The listing builds one solid part. Answer for the finished solid, in the listing's coordinates (mm). A direction names the side the tool comes from. Give positions to 0.01 mm unless a question says otherwise; leave off trailing zeros. Write each loop counter-clockwise with the first axis right and the second up, starting at its lowest first coordinate (ties: lowest second). Pieces come first, ordered by that corner, then holes. Notation, with made-up numbers: (86.25, 73) - (141.25, 73) arc R16 ccw to (141.25, 77) - close; hole circle Ø1 at (27.5, 73). An arc over 180 degrees is marked (long way). Use a Markdown table: item, result. Add a question column.
from build123d import *

# Parameters (mm, degrees)
SKETCH2_R          = 1.6
CUT_EXTRUDE1_DEPTH = 2
CUT_EXTRUDE3_DEPTH = 9
CIRPATTERN1_COUNT  = 3
SKETCH5_R          = 2.45
CUT_EXTRUDE4_DEPTH = 8.5
SKETCH6_R          = 0.5
CUT_EXTRUDE5_DEPTH = 8.5
CUT_EXTRUDE6_DEPTH = 8.5


with BuildPart() as part:
    # Sketch1 → Revolve1 (revolve)
    with BuildSketch(Plane.XY):
        with BuildLine():
            Line((0, -13.977445887), (3.15, -13.977445887))
            ThreePointArc((3.15, -13.977445887), (3.220710678, -14.006735209), (3.25, -14.077445887))
            Line((3.25, -14.077445887), (3.25, -15.377445887))
            Line((3.25, -15.377445887), (3.4, -15.377445887))
            ThreePointArc((3.4, -15.377445887), (4.602081528, -15.875364359), (5.1, -17.077445887))
            Line((5.1, -17.077445887), (5.1, -22.177445887))
            ThreePointArc((5.1, -22.177445887), (4.602081528, -23.379527415), (3.4, -23.877445887))
            Line((3.4, -23.877445887), (3.35, -23.877445887))
            Line((3.35, -23.877445887), (3.35, -24.877445887))
            ThreePointArc((3.35, -24.877445887), (3.320710678, -24.948156565), (3.25, -24.977445887))
            Line((3.25, -24.977445887), (0, -24.977445887))
            Line((0, -24.977445887), (0, -13.977445887))
        make_face()
    revolve(axis=Axis((0, 36.866666667, 0), (0, -1, 0)))

    # Sketch2 → Cut-Extrude1 (cut)
    with BuildSketch(Plane(origin=(0, -13.977445887, 0), x_dir=(1, 0, 0), z_dir=(0, 1, 0))):
        Circle(SKETCH2_R)
    extrude(amount=-CUT_EXTRUDE1_DEPTH, mode=Mode.SUBTRACT)

    # Sketch4 → Cut-Extrude3 (cut)
    with BuildSketch(Plane(origin=(0, -15.977445887, 0), x_dir=(1, 0, 0), z_dir=(0, 1, 0))):
        with BuildLine():
            Line((-0.42, 0.319853318), (-0.42, 1.543891188))
            ThreePointArc((-0.42, 1.543891188), (-1.354595532, 0.832929416), (-1.539787712, -0.326656419))
            Line((-1.539787712, -0.326656419), (-0.42, 0.319853318))
        make_face()
    cut_extrude3 = extrude(amount=-CUT_EXTRUDE3_DEPTH, mode=Mode.SUBTRACT)

    # CirPattern1: Cut-Extrude3 ×3 about axis
    cirpattern1_axis = Axis((0, 0, -0.022012107), (0, 1, 0))
    for i in range(1, CIRPATTERN1_COUNT):
        add(cut_extrude3.rotate(cirpattern1_axis, i * 360 / CIRPATTERN1_COUNT), mode=Mode.SUBTRACT)

    # Sketch5 → Cut-Extrude4 (cut)
    with BuildSketch(Plane.XZ.offset(24.977445887)):
        Circle(SKETCH5_R)
    extrude(amount=-CUT_EXTRUDE4_DEPTH, mode=Mode.SUBTRACT)

    # Sketch6 → Cut-Extrude5 (cut)
    with BuildSketch(Plane(origin=(0, 0, 0), x_dir=(0, 0, -1), z_dir=(1, 0, 0))):
        with Locations((-2.1, -18.477445887)):
            Circle(SKETCH6_R)
        with Locations((2.1, -18.477445887)):
            Circle(SKETCH6_R)
    extrude(amount=-CUT_EXTRUDE5_DEPTH, mode=Mode.SUBTRACT)

    # Sketch7 → Cut-Extrude6 (cut)
    with BuildSketch(Plane(origin=(0, 0, 0), x_dir=(0, 0, -1), z_dir=(1, 0, 0))):
        with BuildLine():
            Line((1.502497593, -21.270117784), (-1.5, -21.270117784))
            ThreePointArc((-1.5, -21.270117784), (-1.846335949, -20.923781835), (-1.5, -20.577445887))
            Line((-1.5, -20.577445887), (1.502497593, -20.577445887))
            ThreePointArc((1.502497593, -20.577445887), (1.848833542, -20.923781835), (1.502497593, -21.270117784))
        make_face()
    extrude(amount=-CUT_EXTRUDE6_DEPTH, mode=Mode.SUBTRACT)


solid = part.part
1. The part is cut by section A-A (y = -15). Give the vertices of the cut face in (x, z), and give its area (3 significant figures).
2. Consider L1, parallel to Z at x = 0, y = -21.5; L2, parallel to Y at x = -0.25, z = -1.25. Determine where each line is inside the solid, lowest interval first. Write a range as [from, to].
3. Given P1, Ø5.5, axis at x = 0, z = 0.5, coming from the -Y side; P2, Ø1.5, axis at x = 3.5, y = -23.5, coming from the -Z side; P3, Ø1.5, axis at x = 4, y = -17, coming from the +Z side; P4, Ø3, axis at x = 0, z = 0, coming from the -Y side, each flat-ended and moving along its own axis, determine where each tip first touches the part or whether it passes through.
4. For a pull along X with two mould halves and no side action, classify faces 1 (the cylindrical face through (-3.347, -24.384, 0.147)), 2 (the cylindrical face through (-2.93, -18.67, -2.56)), 3 (the cylindrical face through (2.337, -20.787, 0.736)) as released by +X, released by -X, zero draft, split by the parting line, or undercut.
5. The part is cut by section C-C (y = -23.25). Give the vertices of the cut face in (x, z).
6. The part is cut by section B-B (z = 0). Count the separate pieces of the cut face and the enclosed holes in it, and give its area (3 significant figures).
7. Which of the six approach directions +Z, -Z, +X, -X, +Y, -Y give full straight-line access (tool end or side, diameter ignored) to faces 4 (the flat face through (0, -16.477, 0)), 5 (the cylindrical face through (-2.579, -14.737, -1.978)), 6 (the cylindrical face through (-2.9, -18.5, 2.6))?
Check values:
| question | item | result |
|---|---|---|
| 1 | outline | circle Ø6.5 at (0, 0); hole circle Ø3.2 at (0, 0) |
| 1 | area | 25.1 mm2 |
| 2 | L1 | z = [-5.1, -2.45], [2.45, 5.1] |
| 2 | L2 | y = [-16.48, -15.98] |
| 3 | P1 | stops at y = -24.98 |
| 3 | P2 | stops at z = -3.9 |
| 3 | P3 | stops at z = 3.93 |
| 3 | P4 | stops at y = -16.48 |
| 4 | face 1 | split by the parting line |
| 4 | face 2 | zero draft |
| 4 | face 3 | undercut |
| 5 | outline | circle Ø9.44 at (0, 0); hole circle Ø4.9 at (0, 0) |
| 6 | separate pieces | 4 |
| 6 | enclosed holes | 0 |
| 6 | area | 50.1 mm2 |
| 7 | face 4 | -Y |
| 7 | face 5 | +Y |
| 7 | face 6 | -X |
